Geometry: final body of the model. Coordinates: model frame, mm. A direction names the side the tool comes from. Give positions to 0.01 mm unless a question says otherwise; leave off trailing zeros. Order: outer loops, then holes, each group sorted by start corner. A loop starts at its lowest first (then second) coordinate and runs counter-clockwise, first axis right, second up. Notation, with made-up numbers: (17.5, 10.25) -> (40.5, 10.25) arc R18 ccw to (40.5, 19.25) -> close; hole circle Ø7 at (-30, -21). An arc over 180 degrees is marked (long way). One line per item, written item: value. Start each with the question number.
Autodesk Inventor part; units mm, degrees
ref_plane "YZ Plane" through (0, 0, 0) normal (1, 0, 0) x (0, 1, 0)
ref_plane "XZ Plane" through (0, 0, 0) normal (0, 1, 0) x (-1, 0, 0)
ref_plane "XY Plane" through (0, 0, 0) normal (0, 0, 1) x (1, 0, 0)
sketch "Skizze1" plane through (0, 0, 0) normal (0, 0, 1) x (1, 0, 0)
  circle A0 centre (0, 0) radius 3
  dimension "d0" = 6
extrude "Extrusion1" add sketch "Skizze1" along normal blind 16
chamfer "Fase1" distance 0.5 angle 45 2 edges at (-3, 0, 16) (-3, 0, 0)
sketch "Skizze2" plane through (0, 0, 16) normal (0, 0, 1) x (1, 0, 0)
  circle A0 centre (0, 0) radius 2.5
hole "Bohrung1" at (0, 0, 16) direction (0, 0, -1) diameter 2.459 depth 10 tip angle 118
properties part number "13_0204_021"
1. Access query for faces 4 (the flat face through (1, 1, 16)), 5 (the cylindrical face through (0.748, 0.976, 10.93)). Directions: +Z, -Z, +X, -X, +Y, -Y. A direction counts if a zero-diameter tool reaches every point of the face in a straight line with its end or side. Return the directions, or none.
2. Cut plane A-A, the plane z = 13.75. Return loops of the section in (x, y).
3. Draft query along Z for faces 1 (the cylindrical face through (-3, 0, 8)), 2 (the conical face through (0.064, -0.204, 5.39)), 3 (the flat face through (0, 0, 0)). Return one class per face: pulls with the +Z half, pulls with the -Z half, needs draft (parallel to the pull), parting line crosses it, or undercut.
4. Cut plane B-B, the plane z = 4.75. Return loops of the section in (x, y).
5. Material intervals for L1, parallel to Y at x = 0, z = 11.25; L2, parallel to Z at x = -2.7, y = -0.05; L3, parallel to Y at x = -1.95, z = 11.5, sorted ascending. Write a range as [from, to].
Answers follow:
1. face 4: +Z, +X, -X, +Y, -Y
1. face 5: +Z
2. outline: circle Ø6 at (0, 0); hole circle Ø2.46 at (0, 0)
3. face 1: needs draft
3. face 2: pulls with the +Z half
3. face 3: pulls with the -Z half
4. outline: circle Ø6 at (0, 0)
5. L1: y = [-3, -1.23], [1.23, 3]
5. L2: z = [0.2, 15.8]
5. L3: y = [-2.28, 2.28]
